from build123d import *

# Parameters (mm, degrees)
F0_W     = 15.24
F0_H     = 15.4686
F1_DEPTH = 3.1242


# Not quite as in the source:
# - the program builds the solid bodies; features that only make, move or delete a surface that nothing else refers to are left out


with BuildPart() as f1:
    # F0 (on Front) → F1 (new body)
    with BuildSketch(Plane.XZ):
        Polygon((-7.62, -7.7343), (-7.62, 7.7343), (-9.9592747303, 6.3627), (-20.8109102848, 0), (-9.9592747303, -6.3627), align=None)
        Rectangle(F0_W, F0_H)
        with BuildLine():
            ThreePointArc((7.62, -7.7343), (15.3543, 0), (7.62, 7.7343))
            Line((7.62, 7.7343), (7.62, -7.7343))
        make_face()
        Polygon((-20.8109102848, 0), (-9.9592747303, 6.3627), (-22.6592747303, 6.3627), (-25.0076241791, 6.3627), (-25.0076241791, -6.3627), (-22.6592747303, -6.3627), (-9.9592747303, -6.3627), align=None)
    extrude(amount=F1_DEPTH)


solid = f1.part
Geometry: final body of the model. Coordinates: model frame, mm. A direction names the side the tool comes from. Coordinates: 2 decimals unless noted, no trailing zeros. Loops run counter-clockwise (first coordinate to the right, second up) from the corner with the lowest first, then second, coordinate; pieces in that order, holes last. Notation, with made-up numbers: (56, 76) - (65, 76) arc R16 cw to (65, 87) - close; hole circle Ø7 at (56, 68). An arc over 180 degrees is marked (long way). Put each result on its own line as item: value. Start each with the question number.
Q1. Pin query (flat end, axial travel): pin 1 Ø1.6 at (x, y) = (-20, -2) entering from -Z; pin 2 Ø1.6 at (x, y) = (-14, -2) entering from +Z. Return the tip coordinate at first contact, or that it passes through.
Q2. Cut plane B-B, the plane x = -14. Return loops of the section in (y, z), and give its area (3 significant figures).
Q3. Cut plane C-C, the plane z = 5.5. Return loops of the section in (x, y).
Q4. Cut plane A-A, the plane y = -1.65. Return loops of the section in (x, z).
Q5. Set-up query: faces 1 (the flat face through (-17, -2, 6.363)), 2 (the cylindrical face through (15.352, -1.54, -0.17)), 3 (the flat face through (-18, -2, -6.363)). Return all of +Z, -Z, +X, -X, +Y, -Y with unobstructed straight access to the full face (end or side cutting, diameter ignored); none if empty.
Q6. Line query: line 1 (Z direction, x = -11.5, y = -1.05); line 2 (X direction, y = -0.7, z = 4.25); line 3 (Z direction, x = 11.5, y = -2.9). Output: solid intervals per line, ascending.
Filled sheet:
1. pin 1: z = -6.36
1. pin 2: z = 6.36
2. outline: (-3.12, -6.36) - (0, -6.36) - (0, 6.36) - (-3.12, 6.36) - close
2. area: 39.8 mm²
3. outline: (-25.01, -3.12) - (13.06, -3.12) - (13.06, 0) - (-25.01, 0) - close
4. outline: (-25.01, -6.36) - (-9.96, -6.36) - (-7.62, -7.73) - (7.62, -7.73) arc R7.73 ccw to (7.62, 7.73) - (-7.62, 7.73) - (-9.96, 6.36) - (-25.01, 6.36) - close
5. face 1: +Z, -X, +Y, -Y
5. face 2: +X, +Y, -Y
5. face 3: -Z, -X, +Y, -Y
6. line 1: -6.36 to 6.36
6. line 2: -25.01 to 14.08
6. line 3: -6.69 to 6.69
